Autodesk Inventor part; units mm, degrees
ref_plane "YZ Plane" through (0, 0, 0) normal (1, 0, 0) x (0, 1, 0)
ref_plane "XZ Plane" through (0, 0, 0) normal (0, 1, 0) x (-1, 0, 0)
ref_plane "XY Plane" through (0, 0, 0) normal (0, 0, 1) x (1, 0, 0)
sketch "Sketch1" plane through (0, 0, 0) normal (0, 0, 1) x (1, 0, 0)
  circle A0 centre (0, 0) radius 65
  dimension "d0" = 130
extrude "Extrusion1" add sketch "Sketch1" along normal blind 5.5
sketch "Sketch4" plane through (0, 0, 5.5) normal (0, 0, 1) x (1, 0, 0)
  line L0 (15, -2.7) -> (15, 2.8)
  line L1 (8.6974, 12.6158) -> (22.8395, 26.7579)
  line L2 (22.8395, 26.7579) -> (26.7286, 22.8688)
  line L3 (26.7286, 22.8688) -> (12.5865, 8.7267)
  line L4 (-8.6267, 12.6865) -> (-12.5158, 8.7974)
  line L5 (-12.5158, 8.7974) -> (-26.6579, 22.9395)
  line L6 (-26.6579, 22.9395) -> (-22.7688, 26.8286)
  line L7 (-22.7688, 26.8286) -> (-8.6267, 12.6865)
  line L8 (2.8, 15.1) -> (-2.7, 15.1)
  line L9 (12.5865, 8.7267) -> (8.6974, 12.6158)
  line L10 (-2.7, 15.1) -> (-2.7, 35.1)
  line L11 (-2.7, 35.1) -> (2.8, 35.1)
  line L12 (2.8, 35.1) -> (2.8, 15.1)
  line L13 (-15, 2.9) -> (-15, -2.6)
  line L14 (-35, 2.9) -> (-15, 2.9)
  line L15 (-35, -2.6) -> (-35, 2.9)
  line L16 (-15, -2.6) -> (-35, -2.6)
  line L17 (-12.5865, -8.5267) -> (-8.6974, -12.4158)
  line L18 (-26.7286, -22.6688) -> (-12.5865, -8.5267)
  line L19 (-8.6974, -12.4158) -> (-22.8395, -26.5579)
  line L20 (-22.8395, -26.5579) -> (-26.7286, -22.6688)
  line L21 (15, 2.8) -> (35, 2.8)
  line L22 (35, 2.8) -> (35, -2.7)
  line L23 (35, -2.7) -> (15, -2.7)
  line L24 (-2.8, -14.9) -> (2.7, -14.9)
  line L25 (8.6267, -12.4865) -> (12.5158, -8.5974)
  line L26 (2.7, -14.9) -> (2.7, -34.9)
  line L27 (2.7, -34.9) -> (-2.8, -34.9)
  line L28 (22.7688, -26.6286) -> (8.6267, -12.4865)
  line L29 (12.5158, -8.5974) -> (26.6579, -22.7395)
  line L30 (26.6579, -22.7395) -> (22.7688, -26.6286)
  line L31 (-2.8, -34.9) -> (-2.8, -14.9)
  line L32 (24.2998, 0.05) -> (27.4417, 0.05)
  point P0 (0, 0)
  point P1 (0, 0)
  point P2 (0, 0)
  point P3 (0, 0.1)
  dimension "d21" = 20
  dimension "d22" = 5.5
  dimension "d23" = 360
  dimension "d24" = 2.75
extrude "Extrusion4" cut sketch "Sketch4" against normal blind 10
sketch "Sketch5" plane through (0, 0, 5.5) normal (0, 0, 1) x (1, 0, 0)
  line L0 (54.5, 2.75) -> (60, 2.75)
  line L1 (60, 2.75) -> (60, -2.75)
  line L2 (60, -2.75) -> (54.5, -2.75)
  line L3 (54.5, -2.75) -> (54.5, 2.75)
  line L4 (36.5928, 40.4819) -> (40.4819, 44.371)
  line L5 (40.4819, 44.371) -> (44.371, 40.4819)
  line L6 (44.371, 40.4819) -> (40.4819, 36.5928)
  line L7 (40.4819, 36.5928) -> (36.5928, 40.4819)
  line L8 (-2.75, 54.5) -> (-2.75, 60)
  line L9 (-2.75, 60) -> (2.75, 60)
  line L10 (2.75, 60) -> (2.75, 54.5)
  line L11 (2.75, 54.5) -> (-2.75, 54.5)
  line L12 (-40.4819, 36.5928) -> (-44.371, 40.4819)
  line L13 (-44.371, 40.4819) -> (-40.4819, 44.371)
  line L14 (-40.4819, 44.371) -> (-36.5928, 40.4819)
  line L15 (-36.5928, 40.4819) -> (-40.4819, 36.5928)
  line L16 (-54.5, -2.75) -> (-60, -2.75)
  line L17 (-60, -2.75) -> (-60, 2.75)
  line L18 (-60, 2.75) -> (-54.5, 2.75)
  line L19 (-54.5, 2.75) -> (-54.5, -2.75)
  line L20 (-36.5928, -40.4819) -> (-40.4819, -44.371)
  line L21 (-40.4819, -44.371) -> (-44.371, -40.4819)
  line L22 (-44.371, -40.4819) -> (-40.4819, -36.5928)
  line L23 (-40.4819, -36.5928) -> (-36.5928, -40.4819)
  line L24 (2.75, -54.5) -> (2.75, -60)
  line L25 (2.75, -60) -> (-2.75, -60)
  line L26 (-2.75, -60) -> (-2.75, -54.5)
  line L27 (-2.75, -54.5) -> (2.75, -54.5)
  line L28 (40.4819, -36.5928) -> (44.371, -40.4819)
  line L29 (44.371, -40.4819) -> (40.4819, -44.371)
  line L30 (40.4819, -44.371) -> (36.5928, -40.4819)
  line L31 (36.5928, -40.4819) -> (40.4819, -36.5928)
  point P0 (0, 0)
  dimension "d30" = 5.5
  dimension "d31" = 5.5
  dimension "d34" = 360
extrude "Extrusion5" cut sketch "Sketch5" against normal blind 10
properties part number "base"
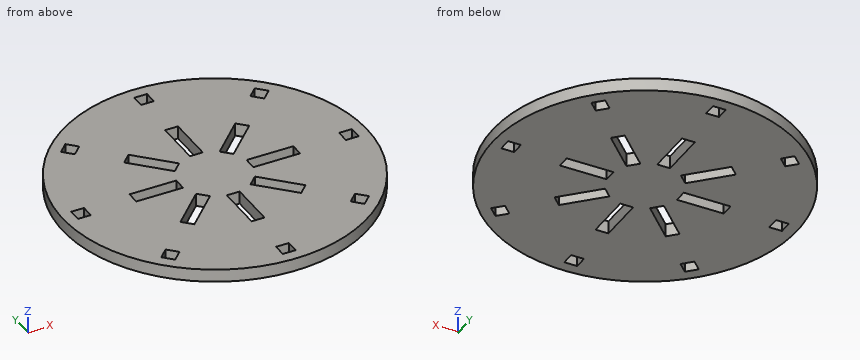
Design review of the part built by this model. Coordinates are the model's own, in mm. Round coordinates to 2 decimals unless told otherwise and drop trailing zeros. Write each loop counter-clockwise with the first axis right and the second up, starting at its lowest first coordinate (ties: lowest second). Pieces come first, ordered by that corner, then holes. Notation, with made-up numbers: (-26.75, -17.5) - (12.25, -17.5) arc R11 cw to (12.25, -9.5) - close; hole circle Ø2 at (47.25, -7.75). An arc over 180 degrees is marked (long way). Return JSON: item names as keys, results as strings. Group by question number.
Item 1: We need section B-B on y = 0. Write out the cut boundary in (x, z).
Item 2: Insertion check: P1, Ø3, axis at x = -25, z = 1.5, coming from the +Y side; P2, Ø3, axis at x = 22, z = 2, coming from the -Y side; P3, Ø3, axis at x = 50, z = 2, coming from the +Y side. Each pin has a flat end and moves straight along its axis. Give the tip position at first contact, or say it passes through.
Item 3: We need section D-D on z = 4. Give the number of separate pieces and of enclosed holes in the cut face, and give its area (3 significant figures).
Item 4: For probe 1 along Y at (x, z) = (19.5, 2.6); probe 2 along X at (y, z) = (41.5, 4.1); probe 3 along Y at (x, z) = (-26, 2.4), list the stretches that pass through material, from the lowest coordinate up. Write a range as [from, to].
Item 5: We need section A-A on x = 0. Write out the cut boundary in (y, z).
Item 6: We need section C-C on x = 29. Write out the cut boundary in (y, z).
Model answer:
{
 "1": {"outline": "(-65, 0) - (-60, 0) - (-60, 5.5) - (-65, 5.5) - close; (-54.5, 0) - (-35, 0) - (-35, 5.5) - (-54.5, 5.5) - close; (-15, 0) - (15, 0) - (15, 5.5) - (-15, 5.5) - close; (35, 0) - (54.5, 0) - (54.5, 5.5) - (35, 5.5) - close; (60, 0) - (65, 0) - (65, 5.5) - (60, 5.5) - close"},
 "2": {"P1": "stops at y = 60.6", "P2": "stops at y = -61.68", "P3": "stops at y = 43.28"},
 "3": {"separate pieces": "1", "enclosed holes": "16", "area": "12,200 mm²"},
 "4": {"probe 1": "y = [-62.01, -23.36], [-15.58, -2.7], [2.8, 15.64], [23.42, 62.01]", "probe 2": "x = [-50.03, -43.35], [-37.61, 37.61], [43.35, 50.03]", "probe 3": "y = [-59.57, -23.4], [-21.94, -2.6], [2.9, 22.28], [23.6, 59.57]"},
 "5": {"outline": "(-65, 0) - (-60, 0) - (-60, 5.5) - (-65, 5.5) - close; (-54.5, 0) - (-34.9, 0) - (-34.9, 5.5) - (-54.5, 5.5) - close; (-14.9, 0) - (15.1, 0) - (15.1, 5.5) - (-14.9, 5.5) - close; (35.1, 0) - (54.5, 0) - (54.5, 5.5) - (35.1, 5.5) - close; (60, 0) - (65, 0) - (65, 5.5) - (60, 5.5) - close"},
 "6": {"outline": "(-58.17, 0) - (-2.7, 0) - (-2.7, 5.5) - (-58.17, 5.5) - close; (2.8, 0) - (58.17, 0) - (58.17, 5.5) - (2.8, 5.5) - close"}
}
